Verification items for the finished model (mm, model axes). A direction names the side the tool comes from. Round coordinates to 2 decimals unless told otherwise and drop trailing zeros. Write each loop counter-clockwise with the first axis right and the second up, starting at its lowest first coordinate (ties: lowest second). Pieces come first, ordered by that corner, then holes. Notation, with made-up numbers: (70, 4) - (112, 4) arc R12 ccw to (112, 15) - close; hole circle Ø9 at (13, -16). An arc over 180 degrees is marked (long way). Answer as a JSON object with one key per item and string values.
```python
from build123d import *


with BuildPart() as f1:
    # F0 (on Front) → F1 (revolve)
    with BuildSketch(Plane.XZ):
        Polygon((-401, -258.865593), (-400, -258.865593), (-400, -162.865593), (-350, -66.865593), (-350, -3.865593), (-351, -3.865593), (-351, 36.134407), (-399, 36.134407), (-399, -3.865593), (-400, -3.865593), (-400, -66.865593), (-450, -162.865593), (-450, -258.865593), (-449, -258.865593), (-449, -218.865593), (-401, -218.865593), align=None)
    revolve(axis=Axis((0, 0, -0.829662), (0, 0, -1)))


solid = f1.part
```
Q1. Section check C-C, the plane z = -144.5. Record the cut outline in (x, y), then the cut area to 3 significant figures.
Geometry check:
{"outline": "circle Ø880.87 at (0, 0); hole circle Ø780.87 at (0, 0)", "area": "131,000 mm2"}
Q2. Set-up check for faces 1 (the cylindrical face through (-380.575, 119.849, 15.854)), 2 (the cylindrical face through (257.96, 236.55, -34.92)), 3 (the cylindrical face through (-382.5, 120.4, -239.1)): record each of +Z, -Z, +X, -X, +Y, -Y from which the full face is reachable in a straight line by a thin tool's end or side.
Geometry check:
{"face 1": "+Z", "face 2": "+Z, -Z", "face 3": "-Z"}
Q3. Gauge pin test, flat ends, axial feed: P1, Ø6, axis at y = -250, z = -140, coming from the +X side; P2, Ø5, axis at x = 114, z = -214.5, coming from the -Y side; P3, Ø1.5, axis at y = -139, z = -124, coming from the -X side. Record the tip position at first contact, or that the pin passes through.
Geometry check:
{"P1": "stops at x = 362.56", "P2": "stops at y = -435.97", "P3": "stops at x = -407.14"}
Q4. Material ranges on line 1 along Y through (x, z) = (0, -243.5); line 2 along X through (y, z) = (297, -220); line 3 along X through (y, z) = (-3.5, -216), recorded low to high. Write a range as [from, to].
Geometry check:
{"line 1": "y = [-450, -449], [-401, -400], [400, 401], [449, 450]", "line 2": "x = [-338.07, -336.74], [-269.43, -267.94], [267.94, 269.43], [336.74, 338.07]", "line 3": "x = [-449.99, -399.98], [399.98, 449.99]"}
Q5. Release check for a two-part mould opening along Y. For faces 4 (the cylindrical face through (-381.53, 120.15, -35.81)), 5 (the cylindrical face through (58.45, 445.18, -238.59)), 6 (the flat face through (-2, -353, 36.134)), 7 (the cylindrical face through (76.09, -342.653, 16.414)) record: released by +Y, released by -Y, zero draft, split by the parting line, or undercut.
Geometry check:
{"face 4": "split by the parting line", "face 5": "undercut", "face 6": "zero draft", "face 7": "undercut"}
